The listing builds one solid part. Answer for the finished solid, in the listing's coordinates (mm). A direction names the side the tool comes from. Coordinates: 2 decimals unless noted, no trailing zeros. Write each loop counter-clockwise with the first axis right and the second up, starting at its lowest first coordinate (ties: lowest second). Pieces come first, ordered by that corner, then holes. Notation, with made-up numbers: M 46.5,7.25 L 101.5,7.25 A25 cw 101.5,44.25 Z; hole C 34.5,69 d5. An arc over 180 degrees is marked long. Answer as a JSON object with one key per item and string values. Group by question number.
Autodesk Inventor part; units mm, degrees
ref_plane "YZ Plane" through (0, 0, 0) normal (1, 0, 0) x (0, 1, 0)
ref_plane "XZ Plane" through (0, 0, 0) normal (0, 1, 0) x (-1, 0, 0)
ref_plane "XY Plane" through (0, 0, 0) normal (0, 0, 1) x (1, 0, 0)
sketch "Sketch1" plane through (0, 0, 0) normal (0, 0, 1) x (1, 0, 0)
  line L0 (-25, -5) -> (25, -5)
  line L1 (25, -5) -> (25, 5)
  line L2 (25, 5) -> (-25, 5)
  line L3 (-25, 5) -> (-25, -5)
  line L4 (-25, -5) -> (25, 5) construction
  line L5 (25, -5) -> (-25, 5) construction
  line L6 (-25, 5) -> (-13.75, 29)
  line L7 (-13.75, 29) -> (-5.75, 29)
  line L8 (-5.75, 29) -> (25, 5)
  line L9 (-9.75, 29) -> (-9.75, 5) construction
  point P0 (0, 0)
  dimension "d0" = 15.25
  dimension "d1" = 50
  dimension "d2" = 34
  dimension "d3" = 8
  dimension "d4" = 10
extrude "Extrusion1" add sketch "Sketch1" along normal blind 9
sketch "Sketch2" plane through (-25, -5, 0) normal (0, -1, 0) x (1, 0, 0)
  line L0 (0, 0) -> (50, 0)
  line L1 (50, 0) -> (50, 9)
  line L2 (0, 9) -> (50, 9)
  line L3 (0, 0) -> (0, 9)
  point P0 (25, 0)
  point P1 (5, 4.5)
  point P2 (25, 4.5)
  point P3 (45, 4.5)
  point P4 (50, 4.5)
  dimension "d7" = 20
  dimension "d8" = 20
  dimension "d9" = 5
hole "Hole1" at (20, -5, 4.5) at (-20, -5, 4.5) at (0, -5, 4.5) direction (0, 1, 0) diameter 2.9 depth 10
sketch "Sketch3" plane through (-13.75, 29, 0) normal (0, 1, 0) x (1, 0, 0)
  line L0 (8, 0) -> (0, 0)
  line L1 (0, 0) -> (0, -9)
  line L2 (8, -9) -> (0, -9)
  line L3 (8, 0) -> (8, -9)
  point P0 (13.75, 0)
  point P1 (4, -4.5)
  point P2 (8, -4.5)
  point P3 (4, 0)
hole "Hole2" at (-9.75, 29, 4.5) direction (0, -1, 0) diameter 2.9 depth 20
sketch "Sketch4" plane through (0, 0, 9) normal (0, 0, 1) x (1, 0, 0)
  line L0 (-11.2, 9) -> (-11.2, 29)
  line L1 (-21.45, 5) -> (-21.45, -5)
  line L2 (-18.55, 5) -> (-18.55, -5)
  line L3 (18.55, 5) -> (18.55, -5)
  line L4 (-5.75, 29) -> (-13.75, 29)
  line L5 (-13.75, 29) -> (-25, 5)
  line L6 (-25, 5) -> (-25, -5)
  line L7 (-25, -5) -> (25, -5)
  line L8 (25, -5) -> (25, 5)
  line L9 (25, 5) -> (-5.75, 29)
  line L10 (21.45, 5) -> (21.45, -5)
  line L11 (-25, -1) -> (25, -1)
  line L12 (-15, -1) -> (-15, 26.3333)
  line L13 (15, 12.8049) -> (15, -1)
  point P0 (0, 0)
  dimension "d25" = 4
  dimension "d26" = 3.55
  dimension "d27" = 3.55
extrude "Extrusion2" cut sketch "Sketch4" against normal through all contours L11 L6 L5 L12 | L13 L9 L8 L11
fillet "Fillet2" radius 2 4 edges at (-25, -3, 9) (-25, -3, 0) (25, -3, 9) (25, -3, 0)
fillet "Fillet3" radius 5 2 edges at (15, -1, 4.5) (-15, -1, 4.5)
fillet "Fillet4" radius 10 2 edges at (15, 12.8049, 4.5) (-15, 26.3333, 4.5)
equation "\"d27\" = d26"
properties part number "RightLevelBlock" material "ABS Plastic"
Item 1: Consider L1, parallel to X at y = -3.25, z = 4.5; L2, parallel to Z at x = -20, y = -2.7; L3, parallel to Y at x = -21.5, z = 8.75. Determine where each line is inside the solid, lowest interval first. Write a range as from..to.
Item 2: A cutting plane is placed at B-B, the plane x = -9.75. Write down the section's boundary in (y, z).
Item 3: A cutting plane is placed at A-A, the plane z = 4.5. Write down the section's boundary in (x, y).
Item 4: For a pull along Z with two mould halves and no side action, classify faces 5 (the face through (-24.43, -3.03, 0.6)), 6 (the face through (0, 8, 9)), 7 (the face through (18.562, -2.863, 4.689)) as +Z half, -Z half, draft (parallel to the pull), parting line (faces both ways), or undercut.
Item 5: Flat-ended cylindrical pins translate along their axes: pin 1 Ø5 at (y, z) = (24.5, 5) entering from +X; pin 2 Ø4 at (y, z) = (13, 5.5) entering from +X; pin 3 Ø4 at (x, z) = (23.5, 6) entering from +Y. Find the tip coordinate at first contact, or state that the pin passes through.
Item 6: A cutting plane is placed at D-D, the plane y = 7. Write down the section's boundary in (x, z), and give its area (3 significant figures).
Item 7: A tool of negligible diameter and unlimited length cuts with its end or side. For faces 1 (the face through (-8.87, 18.86, 3.35)), 2 (the face through (-14.767, 26.25, 4.437)), 3 (the face through (-0.06, 0.07, 5.95)), 4 (the face through (22, -1, 5)), from which of +Z, -Z, +X, -X, +Y, -Y can it reach the whole face along a straight path? Write none if from no direction.
Item 8: A cutting plane is placed at C-C, the plane y = 10.5. Write down the section's boundary in (x, z).
Answer:
{
 "1": {"L1": "-25..-21.45, -18.55..-1.45, 1.45..18.55, 21.45..25", "L2": "0..3.05, 5.95..9", "L3": "-5..-1"},
 "2": {"outline": "M -5,0 L 29,0 L 29,3.05 L 9,3.05 L 9,5.95 L 29,5.95 L 29,9 L -5,9 Z"},
 "3": {"outline": "M -25,-5 L -21.45,-5 L -21.45,-1 L -25,-1 Z; M -18.55,-5 L -1.45,-5 L -1.45,5 L 1.45,5 L 1.45,-5 L 18.55,-5 L 18.55,-0.79 A5 cw 15,4 L 15,7.92 A10 ccw 11.15,15.81 L -5.75,29 L -8.3,29 L -8.3,9 L -11.2,9 L -11.2,29 L -13.75,29 L -14.05,28.35 A10 ccw -15,24.11 L -15,4 A5 cw -18.55,-0.79 Z; M 21.45,-5 L 25,-5 L 25,-1 L 21.45,-1 Z"},
 "4": {"face 5": "-Z half", "face 6": "+Z half", "face 7": "undercut"},
 "5": {"pin 1": "x = 3.22", "pin 2": "x = 14.52", "pin 3": "y = -1"},
 "6": {"outline": "M -15,0 L 15,0 L 15,9 L -15,9 Z", "area": "270 mm2"},
 "7": {"face 1": "+Y", "face 2": "+Z, -Z, -X, +Y", "face 3": "-Y", "face 4": "+Z, -Z, +X, +Y"},
 "8": {"outline": "M -15,0 L 14.66,0 L 14.66,9 L -15,9 Z; hole C -9.75,4.5 d2.9"}
}
